Geometry check sheet. Reference: the model listing, model coordinates, mm. Give positions to 0.01 mm unless a question says otherwise; leave off trailing zeros. Write each loop counter-clockwise with the first axis right and the second up, starting at its lowest first coordinate (ties: lowest second). Pieces come first, ordered by that corner, then holes. Notation, with made-up numbers: (23.25, 63.5) -> (69.25, 63.5) arc R20 cw to (69.25, 97.5) -> close; hole circle Ø1 at (52, 87.25). An arc over 180 degrees is marked (long way). Use a Markdown table: item, result. Add a question column.
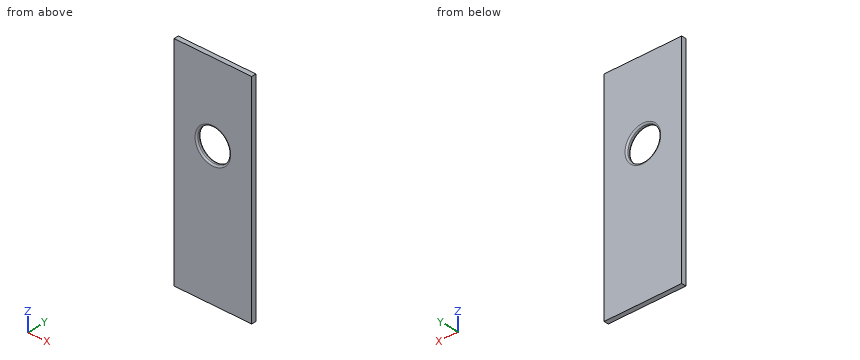
from build123d import *

# Parameters (mm, degrees)
F0_W     = 25
F0_H     = 70
F0_R     = 5.25
F1_DEPTH = 1.5
F2_R     = 0.5


with BuildPart() as f1:
    # F0 (on Front) → F1 (new body)
    with BuildSketch(Plane.XZ):
        Rectangle(F0_W, F0_H)
        with Locations((0, 10)):
            Circle(F0_R, mode=Mode.SUBTRACT)
    extrude(amount=F1_DEPTH)

    # F2
    f2_edges = [f1.edges().sort_by_distance(p)[0] for p in [
        (-5.25, 0, 10),
        (-5.25, -1.5, 10),
    ]]
    fillet(f2_edges, radius=F2_R)


solid = f1.part
1) Sectioned sample at B-B, the plane z = 10. Enter the section's corners in (x, y), and give its area (3 significant figures).
2) Sectioned sample at A-A, the plane x = 0. Enter the section's corners in (y, z), and give its area (3 significant figures).
3) Material ranges on probe 1 along Z at (x, y) = (0, -0.85); probe 2 along Z at (x, y) = (4.75, -0.9); probe 3 along X at (y, z) = (-0.2, 5.5), recorded low to high. Write a range as [from, to].
4) Sectioned sample at C-C, the plane y = -1.25. Enter the section's corners in (x, z), and give its area (3 significant figures).
Check values:
| question | item | result |
|---|---|---|
| 1 | outline | (-12.5, -1.5) -> (-5.75, -1.5) arc R0.5 ccw to (-5.25, -1) -> (-5.25, -0.5) arc R0.5 ccw to (-5.75, 0) -> (-12.5, 0) -> close; (5.25, -1) arc R0.5 ccw to (5.75, -1.5) -> (12.5, -1.5) -> (12.5, 0) -> (5.75, 0) arc R0.5 ccw to (5.25, -0.5) -> close |
| 1 | area | 21.5 mm² |
| 2 | outline | (-1.5, -35) -> (0, -35) -> (0, 4.25) arc R0.5 ccw to (-0.5, 4.75) -> (-1, 4.75) arc R0.5 ccw to (-1.5, 4.25) -> close; (-1.5, 15.75) arc R0.5 ccw to (-1, 15.25) -> (-0.5, 15.25) arc R0.5 ccw to (0, 15.75) -> (0, 35) -> (-1.5, 35) -> close |
| 2 | area | 89.0 mm² |
| 3 | probe 1 | [-35, 4.75], [15.25, 35] |
| 3 | probe 2 | [-35, 7.76], [12.24, 35] |
| 3 | probe 3 | [-12.5, -2.89], [2.89, 12.5] |
| 4 | outline | (-12.5, -35) -> (12.5, -35) -> (12.5, 35) -> (-12.5, 35) -> close; hole circle Ø10.63 at (0, 10) |
| 4 | area | 1,660 mm² |
